```python
from build123d import *

# Parameters (mm, degrees)
BOSS_EXTRUDE1_DEPTH = 3
FILLET1_R           = 1.5
FILLET2_R           = 3
FILLET3_R           = 1.5
FILLET4_R           = 5


with BuildPart() as part:
    # Sketch1 → Boss-Extrude1 (new body)
    with BuildSketch(Plane(origin=(0, 0, 0), x_dir=(1, 0, 0), z_dir=(0, 1, 0))):
        with BuildLine():
            Line((0, 0), (7.31, 0))
            ThreePointArc((7.31, 0), (8.81, -1.5), (7.31, -3))
            Line((7.31, -3), (0, -3))
            ThreePointArc((0, -3), (1.941416089, -7.839258354), (5.823510613, -11.320186386))
            ThreePointArc((5.823510613, -11.320186386), (23.597809929, -16.33), (41.768131919, -13.034040752))
            ThreePointArc((41.768131919, -13.034040752), (42.687342923, -11.923770269), (43.59, -10.8))
            Line((43.59, -10.8), (41.17, -1.78))
            Line((41.17, -1.78), (57.126632367, -3.44))
            ThreePointArc((57.126632367, -3.44), (62.451393238, -1.255638394), (63.57, 4.39))
            ThreePointArc((63.57, 4.39), (63.114921372, 15.71270599), (64.31568295, 26.980755472))
            ThreePointArc((64.31568295, 26.980755472), (63.57, 28), (62.39039615, 27.548959839))
            Line((62.39039615, 27.548959839), (57.126632367, 19.028512497))
            ThreePointArc((57.126632367, 19.028512497), (49.331544712, 11.549647985), (38.89, 8.78))
            ThreePointArc((38.89, 8.78), (34.195061115, 10.662812141), (30.69, 14.31))
            Line((30.69, 14.31), (34.24, 21.27))
            Line((34.24, 21.27), (22.85, 24.35))
            Line((22.85, 24.35), (20.25, 21.818890812))
            Line((20.25, 21.818890812), (20.25, 7.003260248))
            Line((20.25, 7.003260248), (0, 6.204789211))
            Line((0, 6.204789211), (0, 0))
        make_face()
    extrude(amount=BOSS_EXTRUDE1_DEPTH)

    # Fillet1
    fillet1_edges = [part.edges().sort_by_distance(p)[0] for p in [
        (41.17, 1.5, 1.78),
    ]]
    fillet(fillet1_edges, radius=FILLET1_R)

    # Fillet2
    fillet2_edges = [part.edges().sort_by_distance(p)[0] for p in [
        (22.85, 1.5, -24.35),
        (30.69, 1.5, -14.31),
        (38.89, 1.5, -8.78),
        (43.59, 1.5, 10.8),
        (41.768131919, 1.5, 13.034040752),
        (0, 1.5, -6.204789211),
        (20.25, 1.5, -21.818890812),
    ]]
    fillet(fillet2_edges, radius=FILLET2_R)

    # Fillet3
    fillet3_edges = [part.edges().sort_by_distance(p)[0] for p in [
        (34.24, 1.5, -21.27),
    ]]
    fillet(fillet3_edges, radius=FILLET3_R)

    # Fillet4
    fillet4_edges = [part.edges().sort_by_distance(p)[0] for p in [
        (20.25, 1.5, -7.003260248),
    ]]
    fillet(fillet4_edges, radius=FILLET4_R)


solid = part.part
```
Check sheet for the modelled part. Datum: model origin and axes. Units: mm. A direction names the side the tool comes from. Give positions to 0.01 mm unless a question says otherwise; leave off trailing zeros. Write each loop counter-clockwise with the first axis right and the second up, starting at its lowest first coordinate (ties: lowest second). Pieces come first, ordered by that corner, then holes. Notation, with made-up numbers: (-11.75, 45.25) -> (27.25, 45.25) arc R25 cw to (27.25, 82.25) -> close; hole circle Ø11 at (28.5, 50). An arc over 180 degrees is marked (long way). Use CSV: the item, a comma, the result in double quotes. Start each with the question number.
Q1. Cross-section at B-B on x = 44. Enter the section's corners in (y, z).
Q2. Depth check by flat-ended pin: P1, Ø1.5, axis at y = 2, z = -16.5, coming from the -X side; P2, Ø1.5, axis at x = 4, y = 1.5, coming from the -Z side; P3, Ø1.5, axis at x = 33, y = 2.5, coming from the -Z side. Enter the tip coordinate at first touch or a pass-through.
Q3. Cross-section at C-C on z = -5.5. Enter the section's corners in (x, y), and give its area (3 significant figures).
Q4. Tool access check on faces 5 (the cylindrical face through (31.235, 1.521, -14.186)), 6 (the cylindrical face through (49.601, 1.479, -11.703)), 7 (the flat face through (4, 1, 3)), 8 (the cylindrical face through (18.89, 1.52, -8.38)). Record the directions out of +Z, -Z, +X, -X, +Y, -Y that give a thin tool (end or side, any length) a straight path to the whole face; none if there is none.
Q5. Cross-section at A-A on z = -18. Enter the section's corners in (x, y), and give its area (3 significant figures).
Q6. Release check for a two-part mould opening along Z. For faces 1 (the cylindrical face through (8.81, 1.48, 1.47)), 2 (the cylindrical face through (0.82, 1.52, -5.38)), 3 (the flat face through (50.136, 1.479, 2.713)), 4 (the flat face through (32.454, 1.479, -17.768)) record: +Z half, -Z half, draft (parallel to the pull), parting line (faces both ways), or undercut.
Q7. Scan lines: line 1 along Z through (x, y) = (33, 2.5); line 2 along X through (y, z) = (2.5, -13); line 3 along X through (y, z) = (2.75, -17). Record each from-to range of solid material in increasing order.
Working result:
1,outline,"(0, -9.43) -> (3, -9.43) -> (3, 2.07) -> (0, 2.07) -> close"
2,P1,"stops at x = 20.25"
2,P2,"stops at z = -6.39"
2,P3,"stops at z = -21.81"
3,outline,"(0.94, 0) -> (63.45, 0) -> (63.45, 3) -> (0.94, 3) -> close"
3,area,"188 mm^2"
4,face 5,"+Y, -Y"
4,face 6,"-Z, +Y, -Y"
4,face 7,"-X, +Y, -Y"
4,face 8,"-Z, -X, +Y, -Y"
5,outline,"(20.25, 0) -> (32.57, 0) -> (32.57, 3) -> (20.25, 3) -> close; (56.45, 0) -> (63.22, 0) -> (63.22, 3) -> (56.45, 3) -> close"
5,area,"57.3 mm^2"
6,face 1,"undercut"
6,face 2,"-Z half"
6,face 3,"+Z half"
6,face 4,"undercut"
7,line 1,"z = -21.48 to -18.84, -11.58 to 15.69"
7,line 2,"x = 20.25 to 31.67, 51.58 to 63.07"
7,line 3,"x = 20.25 to 32.06, 55.71 to 63.17"
